Build history of the part. All positions in model axes, mm. Face numbers are marked on the shaded views. A direction names the side the tool comes from. Round coordinates to 2 decimals unless told otherwise and drop trailing zeros. Write each loop counter-clockwise with the first axis right and the second up, starting at its lowest first coordinate (ties: lowest second). Pieces come first, ordered by that corner, then holes. Notation, with made-up numbers: (1, 83.25) -> (44, 83.25) arc R13 cw to (44, 98.25) -> close; hole circle Ø5 at (-15.5, 77). An arc over 180 degrees is marked (long way). Answer in a Markdown table with one row per item.
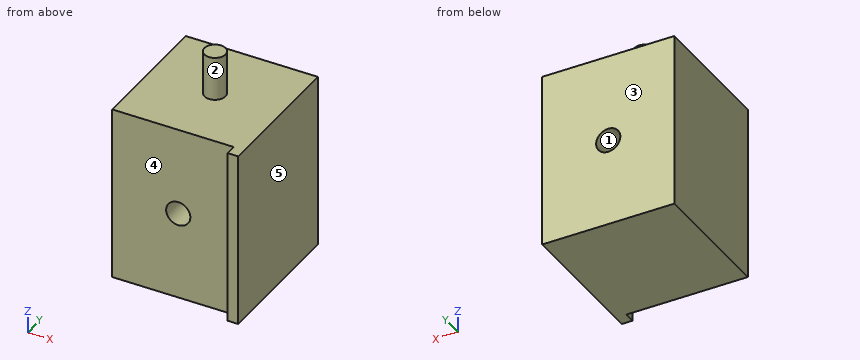
```python
from build123d import *

# Parameters (mm, degrees)
SKETCH1_W           = 38.1
SKETCH1_H           = 38.1
BOSS_EXTRUDE1_DEPTH = 25.4
SKETCH2_R           = 3.048
BOSS_EXTRUDE2_DEPTH = 12.7
SKETCH3_W           = 3.048
SKETCH3_H           = 50.8
BOSS_EXTRUDE3_DEPTH = 3.175
SKETCH4_R           = 3.4925
CUT_EXTRUDE1_DEPTH  = 58.15


with BuildPart() as part:
    # Sketch1 → Boss-Extrude1 (new, symmetric)
    with BuildSketch(Plane.XY):
        Rectangle(SKETCH1_W, SKETCH1_H)
    extrude(amount=BOSS_EXTRUDE1_DEPTH, both=True)

    # Sketch2 → Boss-Extrude2 (add)
    with BuildSketch(Plane.XY.offset(25.4)):
        with Locations(Location((0, 0, 0), (0, 0, 180))):
            Circle(SKETCH2_R)
    extrude(amount=BOSS_EXTRUDE2_DEPTH)

    # Sketch3 → Boss-Extrude3 (add)
    with BuildSketch(Plane.XZ.offset(19.05)):
        with Locations((17.526, 0)):
            Rectangle(SKETCH3_W, SKETCH3_H)
    extrude(amount=BOSS_EXTRUDE3_DEPTH)

    # Sketch4 → Cut-Extrude1 (cut, through all)
    with BuildSketch(Plane.XZ.offset(19.05)):
        with Locations(Location((0, 0, 0), (0, 0, 270))):
            Circle(SKETCH4_R)
    extrude(amount=-CUT_EXTRUDE1_DEPTH, mode=Mode.SUBTRACT)


solid = part.part
```
Q1. Two-plate mould, pull along X, no slides. Class the marked faces 1, 2 and 3: released by +X, released by -X, zero draft, split by the parting line, or undercut.
A:
| item | result |
|---|---|
| face 1 | undercut |
| face 2 | split by the parting line |
| face 3 | zero draft |
Q2. Saw through at D-D on z = 30.5. Write the cut outline in (x, y), plus the area to 3 significant figures.
A:
| item | result |
|---|---|
| outline | circle Ø6.1 at (0, 0) |
| area | 29.2 mm² |
Q3. Which spindle directions (+Z, -Z, +X, -X, +Y, -Y) get a long thin tool onto all of the face, cutting with end or side? Do the marked faces 4 and 5. Say none if no direction does.
A:
| item | result |
|---|---|
| face 4 | +Z, -Z, -X, -Y |
| face 5 | +Z, -Z, +X, +Y, -Y |
Q4. Saw through at C-C on x = 0. Write the cut outline in (y, z).
A:
| item | result |
|---|---|
| outline | (-19.05, -25.4) -> (19.05, -25.4) -> (19.05, -3.49) -> (-19.05, -3.49) -> close; (-19.05, 3.49) -> (19.05, 3.49) -> (19.05, 25.4) -> (3.05, 25.4) -> (3.05, 38.1) -> (-3.05, 38.1) -> (-3.05, 25.4) -> (-19.05, 25.4) -> close |
Q5. Wall check: line 1 (X direction, y = 7, z = 0); line 2 (Z direction, x = -9.5, y = 16.5); line 3 (Y direction, x = 1, z = 16). Give the ranges that are in metal, low to high. Write a range as [from, to].
A:
| item | result |
|---|---|
| line 1 | [-19.05, -3.49], [3.49, 19.05] |
| line 2 | [-25.4, 25.4] |
| line 3 | [-19.05, 19.05] |
Q6. Drop flat-ended pins along their axis: P1, Ø10.5, axis at x = 6.5, z = -10.5, coming from the -Y side; P2, Ø9, axis at x = 0, z = 0, coming from the +Y side; P3, Ø1.6, axis at y = -20, z = 6, coming from the -X side. Give the stop position or say it passes through.
A:
| item | result |
|---|---|
| P1 | y = -19.05 |
| P2 | y = 19.05 |
| P3 | x = 16 |
